The listing builds one solid part. Answer for the finished solid, in the listing's coordinates (mm). A direction names the side the tool comes from. Coordinates: 2 decimals unless noted, no trailing zeros. Loops run counter-clockwise (first coordinate to the right, second up) from the corner with the lowest first, then second, coordinate; pieces in that order, holes last. Notation, with made-up numbers: M 65,54.25 L 89,54.25 A11 ccw 89,70.25 Z; hole C 20.5,86 d1. An arc over 180 degrees is marked long. Return JSON: item names as keys, results as strings. Group by question number.
1. Given P1, Ø1, axis at y = 1, z = 19, coming from the +X side; P2, Ø3, axis at x = -5, y = 1.5, coming from the -Z side; P3, Ø3, axis at y = 0.5, z = 2, coming from the -X side, each flat-ended and moving along its own axis, determine where each tip first touches the part or whether it passes through.
2. Section B-B (z = 0) is taken. Write down the section's boundary in (x, y) (3 decimals).
3. Section D-D (z = -9) is taken. Write down the section's boundary in (x, y), then the cut area to 3 significant figures.
4. The mould has two halves that part along Z. Classify faces 1 (the face through (29.464, 0, 8)), 2 (the face through (18, 0, -12.7)), 3 (the face through (34.798, 0, 25)), 4 (the face through (4.064, 0, 15)): pulls with the +Z half, pulls with the -Z half, needs draft (parallel to the pull), parting line crosses it, or undercut.
5. Straight lines are drawn through the part: L1, parallel to X at y = 1.25, z = 0 (3 decimals); L2, parallel to Z at x = 31.5, y = 0.5; L3, parallel to X at y = 0, z = 18. For each, find the intervals that lie inside material, in ascending order. Write a range as from..to.
6. Section A-A (y = -0.75) is taken. Write down the section's boundary in (x, z) (3 decimals), then the cut area to 3 significant figures.
7. Section C-C (z = 14) is taken. Write down the section's boundary in (x, y).
8. Which of the six approach directions +Z, -Z, +X, -X, +Y, -Y give full straight-line access (tool end or side, diameter ignored) to faces 5 (the face through (12, 3.048, 8)), 6 (the face through (32, 0, -5.08)), 7 (the face through (8, 0, 12.192))?
```python
from build123d import *

# Parameters (mm, degrees)
SKETCH1_R           = 3.175
SKETCH1_W           = 8.89
SKETCH1_H           = 6.096
BOSS_EXTRUDE1_DEPTH = 3.048


with BuildPart() as part:
    # Sketch1 → Boss-Extrude1 (new, symmetric)
    with BuildSketch(Plane(origin=(0, 0, 0), x_dir=(1, 0, 0), z_dir=(0, 1, 0))):
        with BuildLine():
            Line((29.464, -21.59), (29.464, 5.08))
            Line((29.464, 5.08), (34.798, 5.08))
            Line((34.798, 5.08), (34.798, 12.7))
            Line((34.798, 12.7), (0.169222866, 12.7))
            ThreePointArc((0.169222866, 12.7), (-6.521515016, 10.185889524), (-9.900982384, 3.887800513))
            ThreePointArc((-9.900982384, 3.887800513), (-3.674965137, -18.386374523), (16.764, -29.21))
            Line((16.764, -29.21), (34.798, -29.21))
            Line((34.798, -29.21), (34.798, -21.59))
            Line((34.798, -21.59), (29.464, -21.59))
        make_face()
        Circle(SKETCH1_R, mode=Mode.SUBTRACT)
        with Locations((8.509, -15.24)):
            Rectangle(SKETCH1_W, SKETCH1_H, mode=Mode.SUBTRACT)
    extrude(amount=BOSS_EXTRUDE1_DEPTH, both=True)


solid = part.part
```
Worked out:
{
 "1": {"P1": "x = 29.46", "P2": "z = -12.01", "P3": "x = -10.16"},
 "2": {"outline": "M -10.16,-3.048 L -3.175,-3.048 L -3.175,3.048 L -10.16,3.048 Z; M 3.175,-3.048 L 29.464,-3.048 L 29.464,3.048 L 3.175,3.048 Z"},
 "3": {"outline": "M -7.67,-3.05 L 34.8,-3.05 L 34.8,3.05 L -7.67,3.05 Z", "area": "259 mm^2"},
 "4": {"face 1": "undercut", "face 2": "pulls with the -Z half", "face 3": "needs draft", "face 4": "undercut"},
 "5": {"L1": "-10.16..-3.175, 3.175..29.464", "L2": "-12.7..-5.08, 21.59..29.21", "L3": "-3.98..4.06, 12.95..29.46"},
 "6": {"outline": "M -9.901,-3.888 A10.16 ccw 0.169,-12.7 L 34.798,-12.7 L 34.798,-5.08 L 29.464,-5.08 L 29.464,21.59 L 34.798,21.59 L 34.798,29.21 L 16.764,29.21 A29.307 ccw Z; hole C 0,0 d6.35; hole M 4.064,12.192 L 12.954,12.192 L 12.954,18.288 L 4.064,18.288 Z", "area": "1,450 mm^2"},
 "7": {"outline": "M -6.6,-3.05 L 4.06,-3.05 L 4.06,3.05 L -6.6,3.05 Z; M 12.95,-3.05 L 29.46,-3.05 L 29.46,3.05 L 12.95,3.05 Z"},
 "8": {"face 5": "+Z, -Z, +X, -X, +Y", "face 6": "+X, +Y, -Y", "face 7": "+Y, -Y"}
}
